The figure shows three views and two pictorial views of one solid part (mm, origin at its lowest corner). Answer the questions. Give positions to 0.01 mm unless a question says otherwise; leave off trailing zeros. Write each loop counter-clockwise with the first axis right and the second up, starting at its lowest first coordinate (ties: lowest second). Pieces come first, ordered by that corner, then holes. Notation, with made-up numbers: (40.5, 46) -> (55.5, 46) arc R25 cw to (55.5, 78) -> close; hole circle Ø3 at (-7.75, 65.25). An arc over 180 degrees is marked (long way). Write item = value, one per line. Start each with the question number.
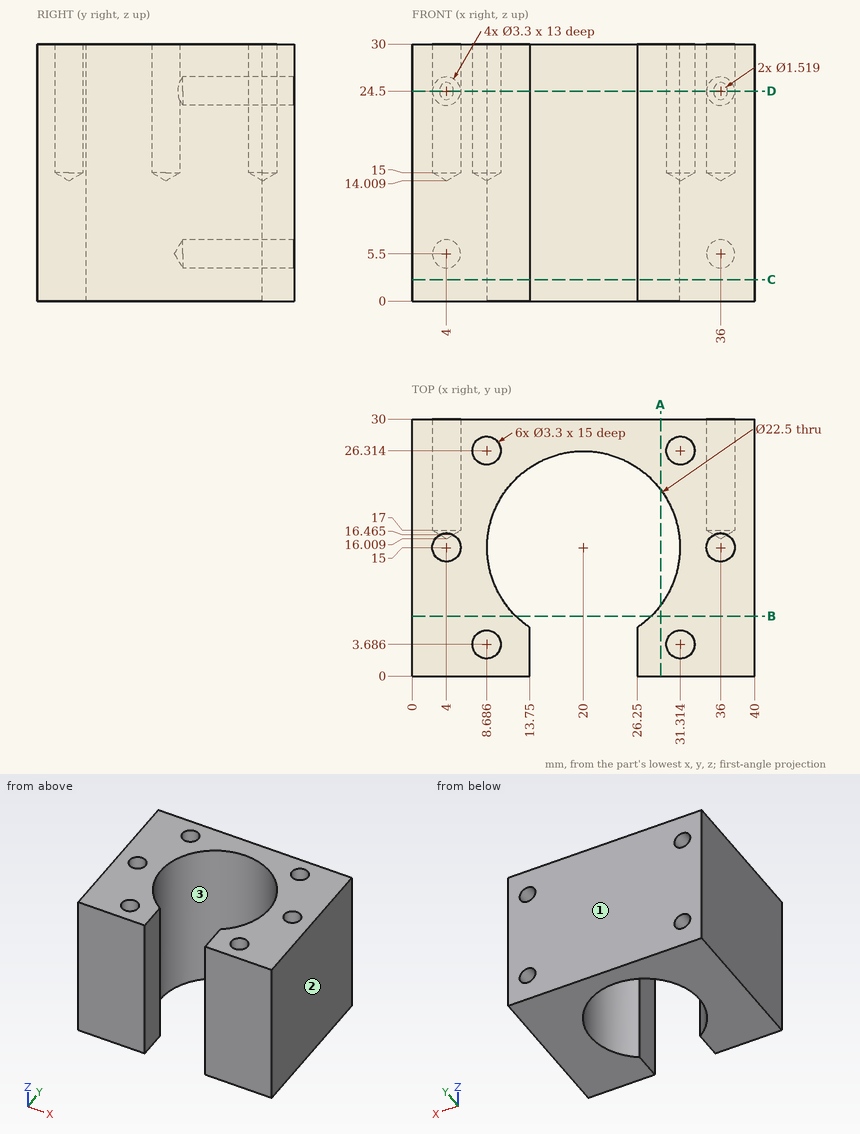
(1) A cutting plane is placed at B-B, the plane y = 7. Write down the section's boundary in (x, z).
(2) A cutting plane is placed at C-C, the plane z = 2.5. Write down the section's boundary in (x, y).
(3) A cutting plane is placed at D-D, the plane z = 24.5. State how many separate pieces and enclosed holes the cut face has.
(4) Find the intervals of material crossed by line 1 along X through (y, z) = (15, 15.5); line 2 along Z through (x, y) = (36, 24.5); line 3 along X through (y, z) = (26.75, 23) (1 decimal), in increasing order.
(5) A cutting plane is placed at A-A, the plane x = 29. Write down the section's boundary in (y, z).
(6) Each of these flat-tipped pins is pushed along its axis until it touches: pin 1 (3 mm diameter, centred on x = 36, z = 24.5, fed in from +Y); pin 2 (3 mm diameter, centred on x = 31.31, y = 26.31, fed in from +Z); pin 3 (2 mm diameter, centred on x = 8.69, y = 26.31, fed in from +Z). Where does it stop, or does it pass through?
(7) Determine the mould class of the marked faces 1, 2 and 3 for opening direction Y: pulls with the +Y half, pulls with the -Y half, needs draft (parallel to the pull), parting line crosses it, or undercut.
Results list:
q1.outline = (0, 0) -> (12.09, 0) -> (12.09, 30) -> (0, 30) -> close; (27.91, 0) -> (40, 0) -> (40, 30) -> (27.91, 30) -> close
q2.outline = (0, 0) -> (13.75, 0) -> (13.75, 5.65) arc R11.25 cw (long way) to (26.25, 5.65) -> (26.25, 0) -> (40, 0) -> (40, 30) -> (0, 30) -> close
q3.separate_pieces = 1
q3.enclosed_holes = 4
q4.line_1 = 0 to 2.35, 5.65 to 8.75, 31.25 to 34.35, 37.65 to 40
q4.line_2 = 0 to 3.85, 7.15 to 22.85, 26.15 to 30
q4.line_3 = 0 to 3.3, 4.7 to 7.1, 10.3 to 29.7, 32.9 to 35.3, 36.7 to 40
q5.outline = (0, 0) -> (8.25, 0) -> (8.25, 30) -> (0, 30) -> close; (21.75, 0) -> (30, 0) -> (30, 30) -> (21.75, 30) -> close
q6.pin_1 = 16.91
q6.pin_2 = 14.91
q6.pin_3 = 14.61
q7.face_1 = pulls with the +Y half
q7.face_2 = needs draft
q7.face_3 = undercut
